from build123d import *

# Parameters (mm, degrees)
SKETCH1_R           = 3.7592
SKETCH1_W           = 1.5875
SKETCH1_H           = 1.3208
BOSS_EXTRUDE1_DEPTH = 1.5875


with BuildPart() as part:
    # Sketch1 → Boss-Extrude1 (new body)
    # profile 1 of 6: a face of its own
    with BuildSketch(Plane.XY):
        with BuildLine():
            ThreePointArc((2.54, 21.59), (-3.139612663, 20.249225326), (-7.62, 16.51))
            ThreePointArc((-7.62, 16.51), (-9.508277885, 12.906092628), (-10.16, 8.89))
            Line((-10.16, 8.89), (-10.16, 4.318))
            Line((-10.16, 4.318), (-10.16, -0.889))
            Line((-10.16, -0.889), (-10.16, -2.2098))
            Line((-10.16, -2.2098), (-10.16, -3.81))
            Line((-10.16, -3.81), (9.525, -3.81))
            Line((9.525, -3.81), (9.525, 0))
            Line((9.525, 0), (9.525, 1.3208))
            Line((9.525, 1.3208), (9.525, 16.51))
            Line((9.525, 16.51), (9.525, 17.8308))
            Line((9.525, 17.8308), (9.525, 21.59))
            Line((9.525, 21.59), (2.54, 21.59))
        make_face()
        Circle(SKETCH1_R, mode=Mode.SUBTRACT)
    # profile 2 of 6: a face of its own
    with BuildSketch(Plane.XY):
        with Locations((-10.95375, -1.5494)):
            Rectangle(SKETCH1_W, SKETCH1_H)
    # profile 3 of 6: a face of its own
    with BuildSketch(Plane.XY):
        with Locations((10.31875, 17.1704)):
            Rectangle(SKETCH1_W, SKETCH1_H)
    # profile 4 of 6: a face of its own
    with BuildSketch(Plane.XY):
        with Locations((10.31875, 0.6604)):
            Rectangle(SKETCH1_W, SKETCH1_H)
    # profile 5 of 6: a face of its own
    with BuildSketch(Plane.XY):
        with BuildLine():
            ThreePointArc((-10.16, 8.89), (-9.508277885, 12.906092628), (-7.62, 16.51))
            Line((-7.62, 16.51), (-17.51946076, 16.51))
            Line((-17.51946076, 16.51), (-22.084921519, 15.561162564))
            Line((-22.084921519, 15.561162564), (-22.084921519, 13.081))
            Line((-22.084921519, 13.081), (-22.084921519, 4.699))
            Line((-22.084921519, 4.699), (-22.084921519, 2.212007412))
            Line((-22.084921519, 2.212007412), (-10.16, 4.318))
            Line((-10.16, 4.318), (-10.16, 8.89))
        make_face()
    # profile 6 of 6: a face of its own
    with BuildSketch(Plane.XY):
        with BuildLine():
            ThreePointArc((-10.16, 8.89), (-9.508277885, 12.906092628), (-7.62, 16.51))
            Line((-7.62, 16.51), (-17.51946076, 16.51))
            Line((-17.51946076, 16.51), (-22.084921519, 15.561162564))
            Line((-22.084921519, 15.561162564), (-22.084921519, 13.081))
            Line((-22.084921519, 13.081), (-22.084921519, 4.699))
            Line((-22.084921519, 4.699), (-22.084921519, 2.212007412))
            Line((-22.084921519, 2.212007412), (-10.16, 4.318))
            Line((-10.16, 4.318), (-10.16, 8.89))
        make_face()
    extrude(amount=BOSS_EXTRUDE1_DEPTH)


solid = part.part
Model file for the job. Use its own axes, mm. A direction names the side the tool comes from. Give positions to 0.01 mm unless a question says otherwise; leave off trailing zeros. Order: outer loops, then holes, each group sorted by start corner. A loop starts at its lowest first (then second) coordinate and runs counter-clockwise, first axis right, second up. Notation, with made-up numbers: (-3, 89) - (21, 89) arc R31 cw to (21, 117) - close; hole circle Ø1 at (48, 21). An arc over 180 degrees is marked (long way). One line per item, written item: value.
Item 1: Slice it at D-D (x = -8). List the corners of the cut face in (y, z), then the cut area to 3 significant figures.
Response values:
outline: (-3.81, 0) - (16.51, 0) - (16.51, 1.59) - (-3.81, 1.59) - close
area: 32.3 mm2
Item 2: Two-plate mould, pull along X, no slides. Class faces 1 (the flat face through (6, 21.59, 1)), 2 (the flat face through (-10.16, 2, 1)), 3 (the flat face through (9.525, 20, 1)), 4 (the flat face through (-16.21, 3.25, 0.78)): released by +X, released by -X, zero draft, split by the parting line, or undercut.
Response values:
face 1: zero draft
face 2: undercut
face 3: released by +X
face 4: undercut
Item 3: Slice it at A-A (z = 0.7). List the corners of the cut face in (x, y) (1 decimal).
Response values:
outline: (-22.1, 2.2) - (-10.2, 4.3) - (-10.2, -0.9) - (-11.7, -0.9) - (-11.7, -2.2) - (-10.2, -2.2) - (-10.2, -3.8) - (9.5, -3.8) - (9.5, 0) - (11.1, 0) - (11.1, 1.3) - (9.5, 1.3) - (9.5, 16.5) - (11.1, 16.5) - (11.1, 17.8) - (9.5, 17.8) - (9.5, 21.6) - (2.5, 21.6) arc R12.7 ccw to (-7.6, 16.5) - (-17.5, 16.5) - (-22.1, 15.6) - close; hole circle Ø7.5 at (0, 0)
Item 4: Wall check: line 1 (X direction, y = 11.5, z = 0.3) (3 decimals); line 2 (Y direction, x = -1, z = 0.25); line 3 (X direction, y = -0.75, z = 1.35) (3 decimals). Give the ranges that are in metal, low to high.
Response values:
line 1: -22.085 to 9.525
line 2: -3.81 to -3.62, 3.62 to 21.09
line 3: -10.16 to -3.684, 3.684 to 9.525
Item 5: Slice it at C-C (y = 12). List the corners of the cut face in (x, z) (1 decimal), then the cut area to 3 significant figures.
Response values:
outline: (-22.1, 0) - (9.5, 0) - (9.5, 1.6) - (-22.1, 1.6) - close
area: 50.2 mm2
Item 6: Pin check, flat tips, straight feed: pin 1 Ø0.8 at (x, z) = (10.5, 0.5) entering from +Y; pin 2 Ø0.8 at (x, z) = (-12.5, 0.5) entering from +Y; pin 3 Ø12 at (x, y) = (0, 0) entering from +Z; pin 4 Ø0.5 at (x, z) = (-10.5, 0.5) entering from -Y. Stop position of each tip, or through.
Response values:
pin 1: y = 17.83
pin 2: y = 16.51
pin 3: z = 1.59
pin 4: y = -2.21
Item 7: Slice it at B-B (x = 0). List the corners of the cut face in (y, z).
Response values:
outline: (-3.81, 0) - (-3.76, 0) - (-3.76, 1.59) - (-3.81, 1.59) - close; (3.76, 0) - (21.33, 0) - (21.33, 1.59) - (3.76, 1.59) - close
Item 8: Tool access for faces 5 (the flat face through (-11, -2.21, 1)), 6 (the flat face through (-11, -0.889, 1)), 7 (the flat face through (-13, 16.51, 1)), 8 (the flat face through (10, 0, 1)), 9 (the flat face through (10, 17.831, 1)): list every direction of +Z, -Z, +X, -X, +Y, -Y with a clear straight run to the whole face (end or side of a thin tool).
Response values:
face 5: +Z, -Z, -X, -Y
face 6: +Z, -Z, -X
face 7: +Z, -Z, -X, +Y
face 8: +Z, -Z, +X, -Y
face 9: +Z, -Z, +X, +Y
